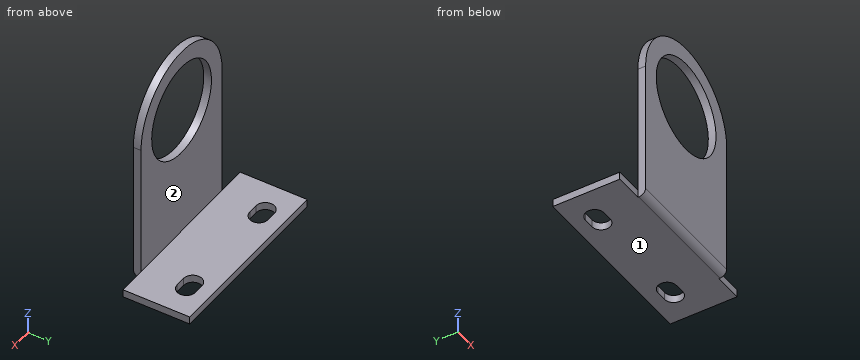
from build123d import *

# Parameters (mm, degrees)
SKETCH_1_R          = 14
EXTRUDE_1_DEPTH     = 2.3
EXTRUDE_2_DEPTH     = 20
FILLET_1_R          = 2
CUT_EXTRUDE_3_DEPTH = 71.530418969


with BuildPart() as part:
    # 草图1 → 拉伸1 (new body)
    with BuildSketch(Plane(origin=(0, 0, 0), x_dir=(1, 0, 0), z_dir=(0, 1, 0))):
        with BuildLine():
            Line((-19, 0), (-19, 42))
            Line((-19, 42), (19, 42))
            Line((19, 42), (19, 0))
            ThreePointArc((19, 0), (0, -19), (-19, 0))
        make_face()
        with Locations(Location((0, 0, 0), (0, 0, 270))):
            Circle(SKETCH_1_R, mode=Mode.SUBTRACT)
    extrude(amount=EXTRUDE_1_DEPTH)

    # 草图2 → 拉伸2 (add)
    with BuildSketch(Plane(origin=(0, 2.3, 0), x_dir=(1, 0, 0), z_dir=(0, 1, 0))):
        Polygon((0, 42), (27.5, 42), (27.5, 39.7), (-27.5, 39.7), (-27.5, 42), align=None)
    extrude(amount=EXTRUDE_2_DEPTH)

    # 圆角1
    fillet_1_edges = [part.edges().sort_by_distance(p)[0] for p in [
        (0, 0, -42),
    ]]
    fillet(fillet_1_edges, radius=FILLET_1_R)

    # 草图3 → 拉伸3 (cut, through all)
    with BuildSketch(Plane(origin=(0, 0, -42), x_dir=(-1, 0, 0), z_dir=(0, 0, -1))):
        with BuildLine():
            Line((-18.5, 18.3), (-15.5, 18.3))
            ThreePointArc((-15.5, 18.3), (-12.75, 15.55), (-15.5, 12.8))
            Line((-15.5, 12.8), (-18.5, 12.8))
            ThreePointArc((-18.5, 12.8), (-21.25, 15.55), (-18.5, 18.3))
        make_face()
        with BuildLine():
            Line((15.5, 18.3), (18.5, 18.3))
            ThreePointArc((18.5, 18.3), (21.25, 15.55), (18.5, 12.8))
            Line((18.5, 12.8), (15.5, 12.8))
            ThreePointArc((15.5, 12.8), (12.75, 15.55), (15.5, 18.3))
        make_face()
    extrude(amount=-CUT_EXTRUDE_3_DEPTH, mode=Mode.SUBTRACT)


solid = part.part
Geometry: final body of the model. Coordinates: model frame, mm. Face numbers are marked on the shaded views. A direction names the side the tool comes from. Round coordinates to 2 decimals unless told otherwise and drop trailing zeros. Loops run counter-clockwise (first coordinate to the right, second up) from the corner with the lowest first, then second, coordinate; pieces in that order, holes last. Notation, with made-up numbers: (83.25, 38.25) -> (114.25, 38.25) arc R20 ccw to (114.25, 47.25) -> close; hole circle Ø10 at (88, 27.5). An arc over 180 degrees is marked (long way). One line per question, with ' | ' between items. Start each with the question number.
1. Line query: line 1 along Z through (x, y) = (-18, 4.5); line 2 along Y through (x, z) = (7.5, -20); line 3 along Z through (x, y) = (-5.5, 1). Output: solid intervals per line, ascending. Write a range as [from, to].
2. Section C-C on z = 7.5. Output: boundary loops of the cut face in (x, y).
3. Set-up query: the marked faces 1 and 2. Return all of +Z, -Z, +X, -X, +Y, -Y with unobstructed straight access to the full face (end or side cutting, diameter ignored); none if empty.
4. Section D-D on x = 6. Output: boundary loops of the cut face in (y, z).
5. Section A-A on y = 15.55. Output: boundary loops of the cut face in (x, z).
6. Contact query for flat-ended pins moving along their axis: pin 1 (1.8 mm diameter, centred on x = 17.5, z = -41, fed in from -Y); pin 2 (0.7 mm diameter, centred on x = -25, z = -40.5, fed in from -Y); pin 3 (4 mm diameter, centred on x = 6.5, z = -35.5, fed in from +Y); pin 4 (17 mm diameter, centred on x = 0, z = 0, fed in from -Y). Output: stop coordinate, or through.
7. Section B-B on x = 0. Output: boundary loops of the cut face in (y, z), and give its area (3 significant figures).
Returned:
1) line 1: z = [-42, -39.7] | line 2: y = [0, 2.3] | line 3: z = [-41.73, -12.87], [12.87, 18.19]
2) outline: (-17.46, 0) -> (-11.82, 0) -> (-11.82, 2.3) -> (-17.46, 2.3) -> close; (11.82, 0) -> (17.46, 0) -> (17.46, 2.3) -> (11.82, 2.3) -> close
3) face 1: -Z, +X, -X, +Y, -Y | face 2: +Z, +X, -X, +Y
4) outline: (0, -40) arc R2 ccw to (2, -42) -> (22.3, -42) -> (22.3, -39.7) -> (2.3, -39.7) -> (2.3, -12.65) -> (0, -12.65) -> close; (0, 12.65) -> (2.3, 12.65) -> (2.3, 18.03) -> (0, 18.03) -> close
5) outline: (-27.5, -42) -> (-21.25, -42) -> (-21.25, -39.7) -> (-27.5, -39.7) -> close; (-12.75, -42) -> (12.75, -42) -> (12.75, -39.7) -> (-12.75, -39.7) -> close; (21.25, -42) -> (27.5, -42) -> (27.5, -39.7) -> (21.25, -39.7) -> close
6) pin 1: stops at y = 0 | pin 2: stops at y = 2.3 | pin 3: stops at y = 2.3 | pin 4: passes through
7) outline: (0, -40) arc R2 ccw to (2, -42) -> (22.3, -42) -> (22.3, -39.7) -> (2.3, -39.7) -> (2.3, -14) -> (0, -14) -> close; (0, 14) -> (2.3, 14) -> (2.3, 19) -> (0, 19) -> close | area: 121 mm2
